```python
from build123d import *

# Parameters (mm, degrees)
BOSS_EXTRUDE1_DEPTH                = 4.7
SKETCH2_R                          = 18
BOSS_EXTRUDE2_DEPTH                = 35.3
F_3_5_3_5_DIAMETER_HOLE1_OUTLINE_R = 1.75
F_3_5_3_5_DIAMETER_HOLE1_DEPTH     = 4.7
SKETCH9_R                          = 11
BOSS_EXTRUDE3_DEPTH                = 2
SKETCH10_R                         = 5
BOSS_EXTRUDE4_DEPTH                = 1
SKETCH11_R                         = 4
BOSS_EXTRUDE5_DEPTH                = 18
CHAMFER1_SIZE                      = 0.5


# Read off the part's stored shape, not the designer's step: Ø3.5 (3.5) Diameter Hole1, Tap Drill for M4x0.7 Tap1
with BuildPart() as part:
    # Sketch1 → Boss-Extrude1 (new body)
    with BuildSketch(Plane.XY):
        Polygon((-21, 17), (-17, 21), (17, 21), (21, 17), (21, -17), (17, -21), (-17, -21), (-21, -17), align=None)
    extrude(amount=BOSS_EXTRUDE1_DEPTH)

    # Sketch2 → Boss-Extrude2 (add)
    with BuildSketch(Plane.XY.offset(4.7)):
        Circle(SKETCH2_R)
    extrude(amount=BOSS_EXTRUDE2_DEPTH)

    # Ø3.5 (3.5) Diameter Hole1 outline → Ø3.5 (3.5) Diameter Hole1 (cut)
    with BuildSketch(Plane.XY):
        with Locations((-15.5, 15.5)):
            Circle(F_3_5_3_5_DIAMETER_HOLE1_OUTLINE_R)
        with Locations((15.5, -15.5)):
            Circle(F_3_5_3_5_DIAMETER_HOLE1_OUTLINE_R)
        with Locations((15.5, 15.5)):
            Circle(F_3_5_3_5_DIAMETER_HOLE1_OUTLINE_R)
        with Locations((-15.5, -15.5)):
            Circle(F_3_5_3_5_DIAMETER_HOLE1_OUTLINE_R)
    extrude(amount=F_3_5_3_5_DIAMETER_HOLE1_DEPTH, mode=Mode.SUBTRACT)

    # Tap Drill for M4x0.7 Tap1 outline → Tap Drill for M4x0.7 Tap1 (revolve, cut)
    with BuildSketch(Plane(origin=(14, 0, 0), x_dir=(1, 0, 0), z_dir=(0, -1, 0))):
        Polygon((0, 40), (0, 31.008579979), (1.65, 32), (1.65, 40), align=None)
    revolve(axis=Axis((14, 0, 0), (0, 0, 1)), mode=Mode.SUBTRACT)

    # Tap Drill for M4x0.7 Tap1 2 outline → Tap Drill for M4x0.7 Tap1 2 (revolve, cut)
    with BuildSketch(Plane(origin=(-14, 0, 0), x_dir=(1, 0, 0), z_dir=(0, -1, 0))):
        Polygon((0, 40), (0, 31.008579979), (1.65, 32), (1.65, 40), align=None)
    revolve(axis=Axis((-14, 0, 0), (0, 0, 1)), mode=Mode.SUBTRACT)

    # Tap Drill for M4x0.7 Tap1 3 outline → Tap Drill for M4x0.7 Tap1 3 (revolve, cut)
    with BuildSketch(Plane.XZ.offset(14)):
        Polygon((0, 40), (0, 31.008579979), (1.65, 32), (1.65, 40), align=None)
    revolve(axis=Axis((0, -14, 0), (0, 0, 1)), mode=Mode.SUBTRACT)

    # Tap Drill for M4x0.7 Tap1 4 outline → Tap Drill for M4x0.7 Tap1 4 (revolve, cut)
    with BuildSketch(Plane.XZ.offset(-14)):
        Polygon((0, 40), (0, 31.008579979), (1.65, 32), (1.65, 40), align=None)
    revolve(axis=Axis((0, 14, 0), (0, 0, 1)), mode=Mode.SUBTRACT)

    # Sketch9 → Boss-Extrude3 (add)
    with BuildSketch(Plane.XY.offset(40)):
        Circle(SKETCH9_R)
    extrude(amount=BOSS_EXTRUDE3_DEPTH)

    # Sketch10 → Boss-Extrude4 (add)
    with BuildSketch(Plane.XY.offset(42)):
        Circle(SKETCH10_R)
    extrude(amount=BOSS_EXTRUDE4_DEPTH)

    # Sketch11 → Boss-Extrude5 (add)
    with BuildSketch(Plane.XY.offset(43)):
        Circle(SKETCH11_R)
    extrude(amount=BOSS_EXTRUDE5_DEPTH)

    # Chamfer1
    chamfer1_edges = [part.edges().sort_by_distance(p)[0] for p in [
        (-4, 0, 61),
    ]]
    chamfer(chamfer1_edges, length=CHAMFER1_SIZE)


solid = part.part
```
Work out the finished part from the listing and answer in its coordinate system (mm). A direction names the side the tool comes from. Round coordinates to 2 decimals unless told otherwise and drop trailing zeros. Loops run counter-clockwise (first coordinate to the right, second up) from the corner with the lowest first, then second, coordinate; pieces in that order, holes last. Notation, with made-up numbers: M -14,68.5 L 35,68.5 A25 ccw 35,88.5 Z; hole C 83.25,64.25 d1. An arc over 180 degrees is marked long. Use CSV: the item, a comma, the result in double quotes.
Q1. The mould has two halves that part along Y. Classify faces 3 (the cylindrical face through (15.524, -0.632, 36.056)), 4 (the flat face through (0, -21, 2)), 5 (the cylindrical face through (-0.867, -3.905, 51.628)): pulls with the +Y half, pulls with the -Y half, needs draft (parallel to the pull), parting line crosses it, or undercut.
Determined:
face 3,"undercut"
face 4,"pulls with the -Y half"
face 5,"parting line crosses it"
Q2. Each of these flat-tipped pins is pushed along its axis until it touches: pin 1 (6 mm diameter, centred on x = -10, z = 34, fed in from +Y); pin 2 (8 mm diameter, centred on y = 12, z = 36, fed in from -X); pin 3 (1.5 mm diameter, centred on y = 7, z = 20.5, fed in from +X). Where does it stop, or does it pass through?
Determined:
pin 1,"y = 16.58"
pin 2,"x = -16.12"
pin 3,"x = 16.88"
Q3. Section B-B, the plane y = 9.5 is taken. Determine the outline of the cut face in (x, z).
Determined:
outline,"M -21,0 L 21,0 L 21,4.7 L 15.29,4.7 L 15.29,40 L 5.55,40 L 5.55,42 L -5.55,42 L -5.55,40 L -15.29,40 L -15.29,4.7 L -21,4.7 Z"
Q4. A tool of negligible diameter and unlimited length cuts with its end or side. For faces 1 (the flat face through (-18.4, 0.3, 4.7)), 2 (the flat face through (0, 21, 2)), from which of +Z, -Z, +X, -X, +Y, -Y can it reach the whole face along a straight path? Write none if from no direction.
Determined:
face 1,"+Z"
face 2,"+Z, -Z, +X, -X, +Y"
Q5. Section A-A, the plane z = 14.5 is taken. Determine the outline of the cut face in (x, y), then the cut area to 3 significant figures.
Determined:
outline,"C 0,0 d36"
area,"1,020 mm2"
Q6. Consider L1, parallel to Y at x = 0, z = 35.5; L2, parallel to Y at x = -15.5, z = 2.4; L3, parallel to Z at x = 13, y = 12.5. Determine where each line is inside the solid, lowest interval first.
Determined:
L1,"-18 to -15.65, -12.35 to 12.35, 15.65 to 18"
L2,"-21 to -17.25, -13.75 to 13.75, 17.25 to 21"
L3,"0 to 4.7"
